Could you check a few things on this model? Use its own coordinates, in mm. A direction names the side the tool comes from. Round coordinates to 2 decimals unless told otherwise and drop trailing zeros. Order: outer loops, then holes, each group sorted by start corner. A loop starts at its lowest first (then second) coordinate and runs counter-clockwise, first axis right, second up. Notation, with made-up numbers: M 41.25,83.5 L 88.25,83.5 A24 ccw 88.25,101.5 Z; hole C 86.25,-13.5 d5. An arc over 180 degrees is marked long. Write each question's results on one line, items separated by ' | '. Start each with the question number.
1. Suppose I cut it at C-C on z = -11. Write out the boundary of the cut face in (x, y) (3 decimals), and give its area (3 significant figures).
2. We'd pull the mould along X, two halves only. Please class faces 3 (the flat face through (12.065, 1, -6)), 4 (the flat face through (6, 0, -6)), 5 (the flat face through (0, 1, -6)): released by +X, released by -X, zero draft, split by the parting line, or undercut.
3. I'm going to push a flat-ended pin straight in: pin 1 (1 mm diameter, centred on x = 3, z = -3.5, fed in from +Y). Where does the tip first touch, or does it pass through?
4. Suppose I cut it at A-A on y = 1.3. Write out the boundary of the cut face in (x, z) (3 decimals).
5. For faces 1 (the flat face through (6, 1, -0.635)), 2 (the flat face through (6.3, 2.543, -6.4)), which set-ups out of +Z, -Z, +X, -X, +Y, -Y let a thin tool reach every point of the face, with its end or its side?
6. Suppose I cut it at B-B on x = 11.75. Write out the boundary of the cut face in (y, z) (3 decimals).
7. Please list where these lines run through material, in increasing order: L1, parallel to Z at x = 6.5, y = 0.75 (3 decimals); L2, parallel to Z at x = 2, y = 1.05 (3 decimals); L3, parallel to X at y = 1.5, z = -9.5 (3 decimals).
from build123d import *

# Parameters (mm, degrees)
SKETCH1_W           = 12.7
SKETCH1_H           = 12.7
BOSS_EXTRUDE1_DEPTH = 2.54
FILLET1_R           = 0.635
SHELL1_START        = 0.635
SHELL1_OUTLINE_W    = 1.905
SHELL1_OUTLINE_H    = 11.43
SHELL1_DEPTH        = 11.43
SKETCH2_R           = 2.54
BOSS_EXTRUDE2_DEPTH = 1.905
BOSS_EXTRUDE3_DEPTH = 0.00254


# Read off the part's stored shape, not the designer's step: Shell1
with BuildPart() as part:
    # Sketch1 → Boss-Extrude1 (new body)
    with BuildSketch(Plane(origin=(0, 0, 0), x_dir=(1, 0, 0), z_dir=(0, 1, 0))):
        with Locations((6.35, 6.35)):
            Rectangle(SKETCH1_W, SKETCH1_H)
    extrude(amount=BOSS_EXTRUDE1_DEPTH)

    # Fillet1
    fillet1_edges = [part.edges().sort_by_distance(p)[0] for p in [
        (0, 1.27, -12.7),
        (12.7, 1.27, -12.7),
        (12.7, 1.27, 0),
        (0, 1.27, 0),
    ]]
    fillet(fillet1_edges, radius=FILLET1_R)

    # Shell1 outline → Shell1 (cut)
    with BuildSketch(Plane.YZ.offset(SHELL1_START)):
        with Locations((0.9525, -6.35)):
            Rectangle(SHELL1_OUTLINE_W, SHELL1_OUTLINE_H)
    extrude(amount=SHELL1_DEPTH, mode=Mode.SUBTRACT)

    # Sketch2 → Boss-Extrude2 (add)
    with BuildSketch(Plane(origin=(0, 1.905, 0), x_dir=(-1, 0, 0), z_dir=(0, -1, 0))):
        with Locations(Location((-6.35, 6.35, 0), (0, 0, 270))):
            Circle(SKETCH2_R)
    extrude(amount=BOSS_EXTRUDE2_DEPTH)

    # Sketch3 → Boss-Extrude3 (add)
    with BuildSketch(Plane(origin=(0, 2.54, 0), x_dir=(1, 0, 0), z_dir=(0, 1, 0))):
        with BuildLine():
            Line((5.573346154, 8.001), (6.209363782, 8.001))
            add(Edge.make_bspline(
                [(6.209363782, 8.001), (6.250920349, 8.000813984), (6.331091677, 8.00045512), (6.446705328, 7.996103418), (6.553364582, 7.988304902), (6.651044933, 7.978667169), (6.739706219, 7.965155443), (6.81945947, 7.949665308), (6.890321237, 7.930793814), (6.95309059, 7.908393613), (7.009424058, 7.88198465), (7.062733687, 7.85385722), (7.111814675, 7.820288125), (7.159144287, 7.784895298), (7.202016608, 7.744297677), (7.243106269, 7.701197093), (7.280673012, 7.653884211), (7.314890906, 7.602931741), (7.345931809, 7.549281068), (7.373051219, 7.492836279), (7.395048965, 7.433508057), (7.413502339, 7.371680187), (7.428324268, 7.307355365), (7.438190216, 7.240137987), (7.444891665, 7.17049739), (7.445482975, 7.123099955), (7.445782051, 7.099127003)],
                knots=[0, 0, 0, 0, 1.698747864, 3.27724071, 4.728299578, 6.070144658, 7.288476769, 8.393259625, 9.389771311, 10.283485332, 11.113357557, 11.931608583, 12.74405601, 13.541433047, 14.344816069, 15.154114104, 15.974336324, 16.810834471, 17.661136416, 18.50621059, 19.367396281, 20.244825668, 21.142564693, 22.063065223, 23.020325768, 24, 24, 24, 24], degree=3))
            add(Edge.make_bspline(
                [(7.445782051, 7.099127003), (7.445349325, 7.072606297), (7.444498965, 7.02048985), (7.436162698, 6.944093533), (7.421921719, 6.871256561), (7.403309504, 6.801364688), (7.377356095, 6.735567789), (7.347705543, 6.672295931), (7.31122596, 6.613323062), (7.269542204, 6.557911502), (7.224018788, 6.50561073), (7.173574986, 6.457930831), (7.11917228, 6.414546773), (7.061125587, 6.375003888), (6.999216983, 6.339381942), (6.933491138, 6.307347374), (6.863499238, 6.279924749), (6.814758985, 6.265582938), (6.790047877, 6.258311699)],
                knots=[0, 0, 0, 0, 1.102006807, 2.165578795, 3.188629044, 4.184801286, 5.166646146, 6.124351954, 7.085497154, 8.042432466, 9.003981491, 9.963833307, 10.922997304, 11.89326795, 12.880200226, 13.889073926, 14.929769137, 16, 16, 16, 16], degree=3))
            add(Edge.make_bspline(
                [(6.790047877, 6.258311699), (6.773771719, 6.254262164), (6.738512321, 6.245489569), (6.680167701, 6.236583183), (6.612931652, 6.228394308), (6.536586757, 6.221356962), (6.451089, 6.216573206), (6.356521166, 6.212837306), (6.252840398, 6.210120921), (6.180744892, 6.210024531), (6.143217949, 6.209974359)],
                knots=[0, 0, 0, 0, 0.618981996, 1.340914327, 2.176866532, 3.120127938, 4.170906482, 5.338178032, 6.614476169, 8, 8, 8, 8], degree=3))
            Line((6.143217949, 6.209974359), (6.143217949, 4.826))
            Line((6.143217949, 4.826), (5.573346154, 4.826))
            Line((5.573346154, 4.826), (5.573346154, 8.001))
        make_face()
        with BuildLine():
            Line((6.143217949, 6.779846154), (6.344835537, 6.779846154))
            add(Edge.make_bspline(
                [(6.344835537, 6.779846154), (6.38152304, 6.780078781), (6.449028591, 6.780506819), (6.541217335, 6.786696491), (6.615301984, 6.796149371), (6.673830231, 6.809706987), (6.720043827, 6.830282464), (6.759900159, 6.854084417), (6.794085953, 6.884181333), (6.823685819, 6.918572209), (6.84735002, 6.958089049), (6.863759911, 7.002088399), (6.874419453, 7.049645784), (6.875403961, 7.082742577), (6.875910256, 7.099763021)],
                knots=[0, 0, 0, 0, 1.8619151, 3.425951444, 4.686033666, 5.651700536, 6.461346321, 7.243864085, 7.999046032, 8.762387399, 9.539336099, 10.322741239, 11.137448474, 12, 12, 12, 12], degree=3))
            add(Edge.make_bspline(
                [(6.875910256, 7.099763021), (6.875409169, 7.114633561), (6.874436938, 7.143485985), (6.867294669, 7.185127188), (6.855911946, 7.22394538), (6.839418817, 7.259535156), (6.818097108, 7.291836043), (6.792101629, 7.320835316), (6.761765954, 7.34715402), (6.73834504, 7.361084912), (6.726446114, 7.36816246)],
                knots=[0, 0, 0, 0, 1.102301479, 2.1387299, 3.123554645, 4.094223062, 5.036071848, 5.982632524, 6.975082478, 8, 8, 8, 8], degree=3))
            add(Edge.make_bspline(
                [(6.726446114, 7.36816246), (6.716367037, 7.373259738), (6.695027566, 7.384051721), (6.658684377, 7.39659819), (6.616744892, 7.407182518), (6.568925973, 7.415967409), (6.515418382, 7.422785396), (6.456231666, 7.427999451), (6.391278727, 7.430096225), (6.346107844, 7.430774724), (6.32257492, 7.431128205)],
                knots=[0, 0, 0, 0, 0.656809284, 1.390599849, 2.23162475, 3.173112763, 4.218524733, 5.370385145, 6.63003504, 8, 8, 8, 8], degree=3))
            Line((6.32257492, 7.431128205), (6.143217949, 7.431128205))
            Line((6.143217949, 7.431128205), (6.143217949, 6.779846154))
        make_face(mode=Mode.SUBTRACT)
    extrude(amount=BOSS_EXTRUDE3_DEPTH)


solid = part.part
Filled sheet:
1) outline: M 0,0 L 0.635,0 L 0.635,1.905 L 12.065,1.905 L 12.065,0 L 12.7,0 L 12.7,2.54 L 0,2.54 Z | area: 10.5 mm^2
2) face 3: undercut | face 4: zero draft | face 5: released by -X
3) pin 1: stops at y = 2.54
4) outline: M 0,-12.065 A0.635 ccw 0.635,-12.7 L 12.065,-12.7 A0.635 ccw 12.7,-12.065 L 12.7,-0.635 A0.635 ccw 12.065,0 L 0.635,0 A0.635 ccw 0,-0.635 Z; C 6.35,-6.35 d5.08; hole M 0.635,-12.065 L 12.065,-12.065 L 12.065,-0.635 L 0.635,-0.635 Z
5) face 1: -Y | face 2: +Z, -Z, +X, -X, +Y
6) outline: M 0,-12.7 L 2.54,-12.7 L 2.54,0 L 0,0 L 0,-0.635 L 1.905,-0.635 L 1.905,-12.065 L 0,-12.065 Z
7) L1: z = -12.7 to -12.065, -8.886 to -3.814, -0.635 to 0 | L2: z = -12.7 to -12.065, -0.635 to 0 | L3: x = 0 to 0.635, 12.065 to 12.7
